Geometry: final body of the model. Coordinates: model frame, mm. Give positions to 0.01 mm unless a question says otherwise; leave off trailing zeros. Loops run counter-clockwise (first coordinate to the right, second up) from the corner with the lowest first, then second, coordinate; pieces in that order, holes last. Notation, with made-up numbers: M -28.5,-16.75 L 20.5,-16.75 A12 ccw 20.5,-6.75 Z; hole C 56.25,36 d2. An arc over 180 degrees is marked long. Put each result on its own line as item: value.
```python
from build123d import *

# Parameters (mm, degrees)
F0_R     = 15.875
F1_DEPTH = 31.75
F3_D     = 12.7
F4_R     = 5.08


with BuildPart() as f1:
    # F0 (on Front) → F1 (new body)
    with BuildSketch(Plane.XZ):
        Circle(F0_R)
    extrude(amount=F1_DEPTH)

    # F3 (through all)
    with Locations(Plane(origin=(0, 0, 0), x_dir=(1, 0, 0), z_dir=(0, 1, 0))):
        with Locations((0, 0)):
            Hole(F3_D / 2)

    # F4
    f4_edges = [f1.edges().sort_by_distance(p)[0] for p in [
        (-15.875, -31.75, 0),
        (-15.875, 0, 0),
    ]]
    fillet(f4_edges, radius=F4_R)


solid = f1.part
```
Item 1: Section D-D on y = -2. Output: boundary loops of the cut face in (x, z).
Output values:
outline: C 0,0 d29.67; hole C 0,0 d12.7
Item 2: Section A-A on x = 0. Output: boundary loops of the cut face in (y, z) (3 decimals), then the cut area to 3 significant figures.
Output values:
outline: M -31.75,-10.795 A5.08 ccw -26.67,-15.875 L -5.08,-15.875 A5.08 ccw 0,-10.795 L 0,-6.35 L -31.75,-6.35 Z; M -31.75,6.35 L 0,6.35 L 0,10.795 A5.08 ccw -5.08,15.875 L -26.67,15.875 A5.08 ccw -31.75,10.795 Z
area: 583 mm²
Item 3: Pin query (flat end, axial travel): pin 1 Ø1 at (x, y) = (12, -25) entering from +Z; pin 2 Ø1.5 at (y, z) = (-19.5, -9) entering from -X; pin 3 Ø6 at (x, y) = (11.5, -9) entering from +Z. Return the tip coordinate at first contact, or that it passes through.
Output values:
pin 1: z = 10.94
pin 2: x = -13.56
pin 3: z = 13.41
Item 4: Section B-B on z = 0. Output: boundary loops of the cut face in (x, y) (3 decimals), then the cut area to 3 significant figures.
Output values:
outline: M -15.875,-26.67 A5.08 ccw -10.795,-31.75 L -6.35,-31.75 L -6.35,0 L -10.795,0 A5.08 ccw -15.875,-5.08 Z; M 6.35,-31.75 L 10.795,-31.75 A5.08 ccw 15.875,-26.67 L 15.875,-5.08 A5.08 ccw 10.795,0 L 6.35,0 Z
area: 583 mm²
Item 5: Line query: probe 1 along Z at (x, y) = (0, -24) (3 decimals); probe 2 along Z at (x, y) = (1, -4); probe 3 along Y at (x, z) = (1, -11). Output: solid intervals per line, ascending. Write a range as [from, to].
Output values:
probe 1: [-15.875, -6.35], [6.35, 15.875]
probe 2: [-15.73, -6.27], [6.27, 15.73]
probe 3: [-31.74, -0.01]
Item 6: Section C-C on y = -24.5. Output: boundary loops of the cut face in (x, z) (3 decimals), then the cut area to 3 significant figures.
Output values:
outline: C 0,0 d31.75; hole C 0,0 d12.7
area: 665 mm²
Item 7: Mould query, pull axis Y, two halves, no side actions, for faces 1 (the flat face through (5, -31.75, -5)), 2 (the cylindrical face through (1.38, -16.1, 6.2)), 3 (the flat face through (5, 0, -5)). Classes: pulls with the +Y half, pulls with the -Y half, needs draft (parallel to the pull), parting line crosses it, or undercut.
Output values:
face 1: pulls with the -Y half
face 2: needs draft
face 3: pulls with the +Y half
